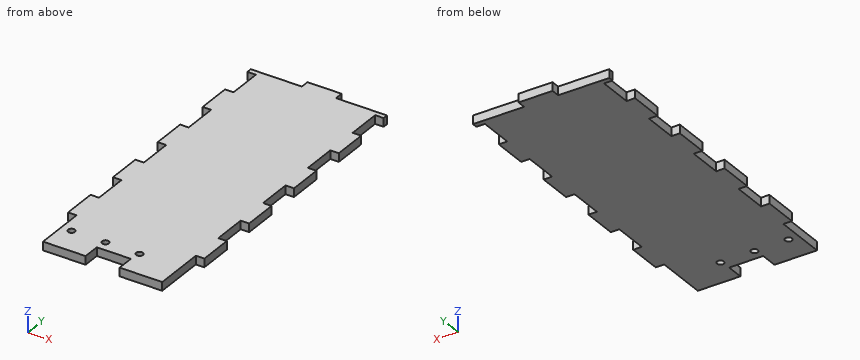
```python
from build123d import *

# Parameters (mm, degrees)
SKETCH_1_W                      = 80
SKETCH_1_H                      = 183
EXTRUDE_1_DEPTH                 = 5
CUT_EXTRUDE_1_REACH             = 101.986
SKETCH_2_W                      = 5
SKETCH_2_H                      = 20
CUT_EXTRUDE_1_DIRECTION_2_DEPTH = 100.986249055
PATTERN_LINEAR_1_COUNT          = 5
PATTERN_LINEAR_1_PITCH          = 40
CUT_EXTRUDE_3_REACH             = 101.986
SKETCH_4_W                      = 5
SKETCH_4_H                      = 20
PATTERN_LINEAR_4_COUNT          = 5
PATTERN_LINEAR_4_PITCH          = 40
SKETCH_5_W                      = 20
SKETCH_5_H                      = 5
EXTRUDE_2_DEPTH                 = 5
SKETCH_6_W                      = 25
SKETCH_6_H                      = 10
EXTRUDE_3_DEPTH                 = 5
CUT_EXTRUDE_4_REACH             = 111.212
SKETCH_7_R                      = 2
PATTERN_LINEAR_5_COUNT          = 2
PATTERN_LINEAR_5_PITCH          = 40
PATTERN_LINEAR_6_COUNT          = 2
PATTERN_LINEAR_6_PITCH          = 20


with BuildPart() as part:
    # 스케치1 → 보스-돌출1 (new body)
    with BuildSketch(Plane.XY):
        Rectangle(SKETCH_1_W, SKETCH_1_H)
    extrude(amount=EXTRUDE_1_DEPTH)

    # 스케치2 → 컷-돌출1 (cut, up to next)
    with BuildSketch(Plane.XY.offset(5), mode=Mode.PRIVATE) as cut_extrude_1_sk1:
        with Locations((-37.5, -81.5)):
            Rectangle(SKETCH_2_W, SKETCH_2_H)
    cut_extrude_1_tool1 = extrude(cut_extrude_1_sk1.sketch, amount=-CUT_EXTRUDE_1_REACH, mode=Mode.PRIVATE) & part.part
    cut_extrude_1 = cut_extrude_1_tool1.solids().sort_by_distance((-37.5, -81.5, 5))[0]
    add(cut_extrude_1, mode=Mode.SUBTRACT)

    # 스케치2 → 컷-돌출1 direction 2 (cut)
    with BuildSketch(Plane.XY.offset(5)):
        with Locations((-37.5, -81.5)):
            Rectangle(SKETCH_2_W, SKETCH_2_H)
    cut_extrude_1_direction_2 = extrude(amount=CUT_EXTRUDE_1_DIRECTION_2_DEPTH, mode=Mode.SUBTRACT)

    # 선형 패턴1: 컷-돌출1, 컷-돌출1 direction 2 ×5
    with Locations(*[(0, i * PATTERN_LINEAR_1_PITCH, 0) for i in range(1, PATTERN_LINEAR_1_COUNT)]):
        add(cut_extrude_1, mode=Mode.SUBTRACT)
        add(cut_extrude_1_direction_2, mode=Mode.SUBTRACT)

    # 스케치4 → 컷-돌출3 (cut, up to next)
    with BuildSketch(Plane.XY.offset(5), mode=Mode.PRIVATE) as cut_extrude_3_sk1:
        with Locations((37.5, -81.5)):
            Rectangle(SKETCH_4_W, SKETCH_4_H)
    cut_extrude_3_tool1 = extrude(cut_extrude_3_sk1.sketch, amount=-CUT_EXTRUDE_3_REACH, mode=Mode.PRIVATE) & part.part
    cut_extrude_3 = cut_extrude_3_tool1.solids().sort_by_distance((37.5, -81.5, 5))[0]
    add(cut_extrude_3, mode=Mode.SUBTRACT)

    # 선형 패턴4: 컷-돌출3 ×5
    with Locations(*[(0, i * PATTERN_LINEAR_4_PITCH, 0) for i in range(1, PATTERN_LINEAR_4_COUNT)]):
        add(cut_extrude_3, mode=Mode.SUBTRACT)

    # 스케치5 → 보스-돌출2 (add)
    with BuildSketch(Plane.XY.offset(5)):
        with Locations((0, 94)):
            Rectangle(SKETCH_5_W, SKETCH_5_H)
    extrude(amount=-EXTRUDE_2_DEPTH)

    # 스케치6 → 보스-돌출3 (add)
    with BuildSketch(Plane.XY.offset(5)):
        with Locations((-22.5, -96.5)):
            Rectangle(SKETCH_6_W, SKETCH_6_H)
        with Locations((22.5, -96.5)):
            Rectangle(SKETCH_6_W, SKETCH_6_H)
    extrude(amount=-EXTRUDE_3_DEPTH)

    # 스케치7 → 컷-돌출4 (cut, up to next)
    with BuildSketch(Plane.XY.offset(5), mode=Mode.PRIVATE) as cut_extrude_4_sk1:
        with Locations((-29, -85.2)):
            Circle(SKETCH_7_R)
    cut_extrude_4_tool1 = extrude(cut_extrude_4_sk1.sketch, amount=-CUT_EXTRUDE_4_REACH, mode=Mode.PRIVATE) & part.part
    cut_extrude_4 = cut_extrude_4_tool1.solids().sort_by_distance((-29, -85.2, 5))[0]
    add(cut_extrude_4, mode=Mode.SUBTRACT)

    # 선형 패턴5: 컷-돌출4 ×2
    with Locations(*[(i * PATTERN_LINEAR_5_PITCH, 0, 0) for i in range(1, PATTERN_LINEAR_5_COUNT)]):
        add(cut_extrude_4, mode=Mode.SUBTRACT)

    # 선형 패턴6: 컷-돌출4 ×2
    with Locations(*[(i * PATTERN_LINEAR_6_PITCH, 0, 0) for i in range(1, PATTERN_LINEAR_6_COUNT)]):
        add(cut_extrude_4, mode=Mode.SUBTRACT)


solid = part.part
```
Read the model definition and answer for the solid it produces. Units are mm, in the model's axes. Coordinates: 2 decimals unless noted, no trailing zeros. Loops run counter-clockwise (first coordinate to the right, second up) from the corner with the lowest first, then second, coordinate; pieces in that order, holes last.
(1) Consider line 1 along Y through (x, z) = (11, 2.65); line 2 along Y through (x, z) = (-9, 3.7); line 3 along Y through (x, z) = (-13.5, 0.5). Determine where each line is inside the solid, lowest interval first.
Solution:
line 1: y = -101.5 to -87.2, -83.2 to 91.5
line 2: y = -91.5 to -87.2, -83.2 to 96.5
line 3: y = -101.5 to 91.5
(2) The part is cut by section A-A (y = -85.2). Determine the outline of the cut face in (x, z).
Solution:
outline: (-35, 0) - (-31, 0) - (-31, 5) - (-35, 5) - close; (-27, 0) - (-11, 0) - (-11, 5) - (-27, 5) - close; (-7, 0) - (9, 0) - (9, 5) - (-7, 5) - close; (13, 0) - (35, 0) - (35, 5) - (13, 5) - close
(3) The part is cut by section C-C (z = 2). Count the separate pieces of the cut face and the enclosed holes in it, and give its area (3 significant figures).
Solution:
separate pieces: 1
enclosed holes: 3
area: 14,200 mm2
(4) The part is cut by section D-D (x = 4). Determine the outline of the cut face in (y, z).
Solution:
outline: (-91.5, 0) - (96.5, 0) - (96.5, 5) - (-91.5, 5) - close
(5) Flat-ended cylindrical pins translate along their axes: pin 1 Ø1.5 at (y, z) = (2, 3) entering from +X; pin 2 Ø2.5 at (x, z) = (37.5, 2) entering from +Y. Find the tip coordinate at first contact, or state that the pin passes through.
Solution:
pin 1: stops at x = 35
pin 2: stops at y = 91.5
(6) The part is cut by section B-B (x = -29). Determine the outline of the cut face in (y, z).
Solution:
outline: (-101.5, 0) - (-87.2, 0) - (-87.2, 5) - (-101.5, 5) - close; (-83.2, 0) - (91.5, 0) - (91.5, 5) - (-83.2, 5) - close
